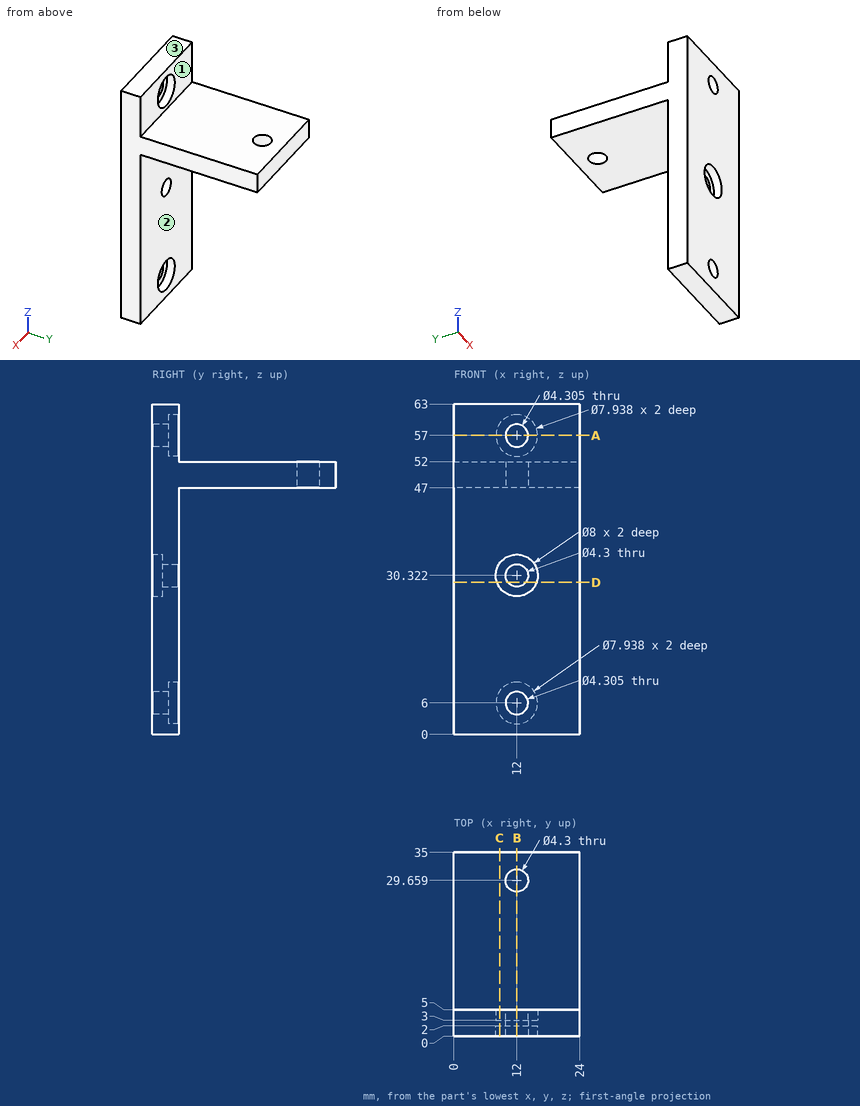
Can you work these out from the drawing? Everything is in mm from the part's minimum corner. A direction names the side the tool comes from. Give positions to 0.01 mm unless a question says otherwise; leave off trailing zeros. Order: outer loops, then holes, each group sorted by start corner. A loop starts at its lowest first (then second) coordinate and runs counter-clockwise, first axis right, second up. Notation, with made-up numbers: (50, 58) -> (60, 58) arc R18 cw to (60, 93) -> close; hole circle Ø9 at (-18, 85.25). An arc over 180 degrees is marked (long way). Return JSON: item names as keys, results as strings.
1. Imagine slicing it at B-B on x = 12. Give the number of separate pieces and of enclosed holes in the cut face, then the cut area to 3 significant figures.
Answer list:
{"separate pieces": "5", "enclosed holes": "0", "area": "357 mm2"}
2. Imagine slicing it at C-C on x = 8.75. List the corners of the cut face in (y, z) for me, then the cut area to 3 significant figures.
Answer list:
{"outline": "(0, 0) -> (5, 0) -> (5, 3.72) -> (3, 3.72) -> (3, 8.28) -> (5, 8.28) -> (5, 47) -> (35, 47) -> (35, 52) -> (5, 52) -> (5, 54.72) -> (3, 54.72) -> (3, 59.28) -> (5, 59.28) -> (5, 63) -> (0, 63) -> (0, 32.65) -> (2, 32.65) -> (2, 27.99) -> (0, 27.99) -> close", "area": "437 mm2"}
3. Imagine slicing it at A-A on z = 57. List the corners of the cut face in (x, y) for me.
Answer list:
{"outline": "(0, 0) -> (9.85, 0) -> (9.85, 3) -> (8.03, 3) -> (8.03, 5) -> (0, 5) -> close; (14.15, 0) -> (24, 0) -> (24, 5) -> (15.97, 5) -> (15.97, 3) -> (14.15, 3) -> close"}
4. Imagine slicing it at D-D on z = 29. List the corners of the cut face in (x, y) for me, then the cut area to 3 significant figures.
Answer list:
{"outline": "(0, 0) -> (8.22, 0) -> (8.22, 2) -> (10.3, 2) -> (10.3, 5) -> (0, 5) -> close; (13.7, 2) -> (15.78, 2) -> (15.78, 0) -> (24, 0) -> (24, 5) -> (13.7, 5) -> close", "area": "94.7 mm2"}
5. I need wall thicknesses on line 1 (Z direction, x = 12, y = 4.05); line 2 (Z direction, x = 12, y = 1.3); line 3 (X direction, y = 3.8, z = 6). Which ranges of each line are inside material? Lowest first, please. Write a range as from..to.
Answer list:
{"line 1": "z = 0..2.03, 9.97..28.17, 32.47..53.03, 60.97..63", "line 2": "z = 0..3.85, 8.15..26.32, 34.32..54.85, 59.15..63", "line 3": "x = 0..8.03, 15.97..24"}
6. On a 3-axis mill with a long thin cutter (end or side, diameter ignored), from which of +Z, -Z, +X, -X, +Y, -Y can I reach the whole of each face in a straight line? I mean the marked faces 1, 2 and 3. Say none if no direction works.
Answer list:
{"face 1": "+Z, +X, -X, +Y", "face 2": "-Z, +X, -X, +Y", "face 3": "+Z, +X, -X, +Y, -Y"}
7. For pin 1 Ø2 at (x, y) = (5, 22) entering from -Z; pin 2 Ø2.5 at (x, z) = (11, 6) entering from +Y; pin 3 Ø3.5 at (x, z) = (12, 30.322) entering from +Y; pin 4 Ø2 at (x, y) = (9.5, 10) entering from +Z, each with a flat end and sliding along its axis, tell me the tip position at first contact or that it passes through.
Answer list:
{"pin 1": "stops at z = 47", "pin 2": "stops at y = 3", "pin 3": "passes through", "pin 4": "stops at z = 52"}
